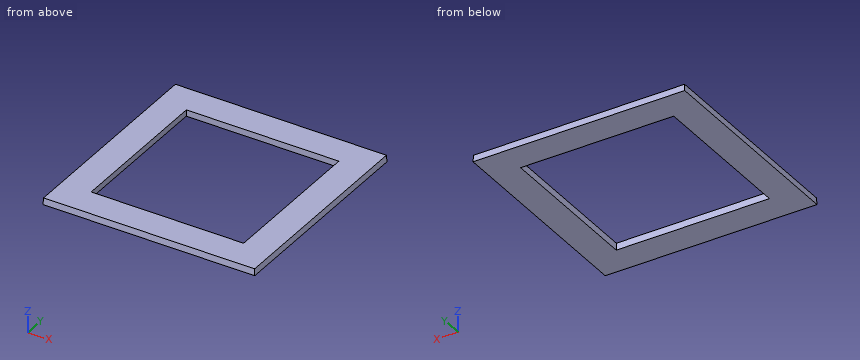
from build123d import *

# Parameters (mm, degrees)
F0_W     = 101.6
F0_H     = 101.6
F1_DEPTH = 3.175
F1_TAPER = 3
F2_T     = -14.0335


# Not quite as in the source:
# - a feature of the source that left no trace in its solid (it failed there, or was rolled back) is left out


with BuildPart() as f1:
    # F0 (on Top) → F1 (new body)
    with BuildSketch(Plane.XY):
        Rectangle(F0_W, F0_H)
    extrude(amount=F1_DEPTH, taper=F1_TAPER)

    # F2
    f2_openings = [f1.faces().sort_by_distance(p)[0] for p in [
        (0, 0, 3.175),
        (0, 0, 0),
    ]]
    offset(amount=F2_T, openings=f2_openings)


solid = f1.part
Work out the finished part from the listing and answer in its coordinate system (mm). Coordinates: 2 decimals unless noted, no trailing zeros. Write each loop counter-clockwise with the first axis right and the second up, starting at its lowest first coordinate (ties: lowest second). Pieces come first, ordered by that corner, then holes. Notation, with made-up numbers: M 43.25,-23 L 99.25,-23 A4 ccw 99.25,-17 Z; hole C 8,53 d2. An arc over 180 degrees is marked long. Answer as CSV lines item,"result". Start each with the question number.
Item 1: Section C-C on z = 0.9 is taken. Write down the section's boundary in (x, y), and give its area (3 significant figures).
Item 2: A flat-ended cylindrical pin translates along its axis: P1, Ø1.5, axis at y = 21, z = 1.5, coming from the +X side. Find the tip coordinate at first contact, or state that the pin passes through.
Item 3: Consider L1, parallel to X at y = 29, z = 0.5; L2, parallel to Y at x = -15, z = 2.9; L3, parallel to Y at x = -5, z = 0.4. Determine where each line is inside the solid, lowest interval first.
Item 4: Section A-A on x = 35 is taken. Write down the section's boundary in (y, z) (3 decimals), and give its area (3 significant figures).
Checks:
1,outline,"M -50.75,-50.75 L 50.75,-50.75 L 50.75,50.75 L -50.75,50.75 Z; hole M -36.7,-36.7 L 36.7,-36.7 L 36.7,36.7 L -36.7,36.7 Z"
1,area,"4,920 mm²"
2,P1,"stops at x = 50.76"
3,L1,"x = -50.77 to -36.72, 36.72 to 50.77"
3,L2,"y = -50.65 to -36.6, 36.6 to 50.65"
3,L3,"y = -50.78 to -36.73, 36.73 to 50.78"
4,outline,"M -50.8,0 L -36.747,0 L -36.581,3.175 L -50.634,3.175 Z; M 36.581,3.175 L 36.747,0 L 50.8,0 L 50.634,3.175 Z"
4,area,"89.2 mm²"
